Part model, mm, in its own coordinate system. A direction names the side the tool comes from. Coordinates: 2 decimals unless noted, no trailing zeros. Loops run counter-clockwise (first coordinate to the right, second up) from the corner with the lowest first, then second, coordinate; pieces in that order, holes last. Notation, with made-up numbers: (77, 27.25) - (124, 27.25) arc R13 ccw to (124, 34.25) - close; hole circle Ø8 at (-18.75, 85). An arc over 180 degrees is marked (long way). Answer as CSV lines item,"result".
from build123d import *

# Parameters (mm, degrees)
SKETCH1_W           = 100
SKETCH1_H           = 56
BOSS_EXTRUDE1_DEPTH = 52
SKETCH4_W           = 44
SKETCH4_H           = 50
CUT_EXTRUDE2_DEPTH  = 126.85706178


with BuildPart() as part:
    # Sketch1 → Boss-Extrude1 (new body)
    with BuildSketch(Plane(origin=(0, 0, 0), x_dir=(1, 0, 0), z_dir=(0, 1, 0))):
        with Locations((50, 28)):
            Rectangle(SKETCH1_W, SKETCH1_H)
    extrude(amount=BOSS_EXTRUDE1_DEPTH)

    # Sketch4 → Cut-Extrude2 (cut, through all)
    with BuildSketch(Plane.ZY):
        with Locations((-28, 31)):
            Rectangle(SKETCH4_W, SKETCH4_H)
    extrude(amount=-CUT_EXTRUDE2_DEPTH, mode=Mode.SUBTRACT)


solid = part.part
Q1. Saw through at B-B (x = 79.5). Give the cut face in (y, z), then the cut area to 3 significant figures.
Results:
outline,"(0, -56) - (52, -56) - (52, -50) - (6, -50) - (6, -6) - (52, -6) - (52, 0) - (0, 0) - close"
area,"888 mm^2"
Q2. Two-plate mould, pull along Z, no slides. Class faces 1 (the face through (49, 26, 0)), 2 (the face through (49, 29, -6)), 3 (the face through (0, 5, -26)): released by +Z, released by -Z, zero draft, split by the parting line, or undercut.
Results:
face 1,"released by +Z"
face 2,"undercut"
face 3,"zero draft"
Q3. Saw through at C-C (z = -19). Give the cut face in (x, y), then the cut area to 3 significant figures.
Results:
outline,"(0, 0) - (100, 0) - (100, 6) - (0, 6) - close"
area,"600 mm^2"
Q4. Saw through at A-A (y = 41.5). Give the cut face in (x, z).
Results:
outline,"(0, -56) - (100, -56) - (100, -50) - (0, -50) - close; (0, -6) - (100, -6) - (100, 0) - (0, 0) - close"
Q5. Wall check: L1, parallel to Z at x = 90, y = 44; L2, parallel to Y at x = 94, z = -40.5. Give the ranges that are in metal, low to high.
Results:
L1,"z = -56 to -50, -6 to 0"
L2,"y = 0 to 6"
Q6. Which spindle directions (+Z, -Z, +X, -X, +Y, -Y) get a long thin tool onto all of the face, cutting with end or side? Do faces 4 (the face through (49, 52, -3)), 5 (the face through (49, 29, -50)). Say none if no direction does.
Results:
face 4,"+Z, -Z, +X, -X, +Y"
face 5,"+X, -X, +Y"
